Print and shaded views of the part. All mm, measured from the part's lowest x, y and z. A direction names the side the tool comes from. Round coordinates to 2 decimals unless told otherwise and drop trailing zeros. Loops run counter-clockwise (first coordinate to the right, second up) from the corner with the lowest first, then second, coordinate; pieces in that order, holes last. Notation, with made-up numbers: (-35, 27.5) - (1, 27.5) arc R19 ccw to (1, 57.5) - close; hole circle Ø2 at (83, 43). An arc over 180 degrees is marked (long way). Put each result on its own line as item: value. Start each with the question number.
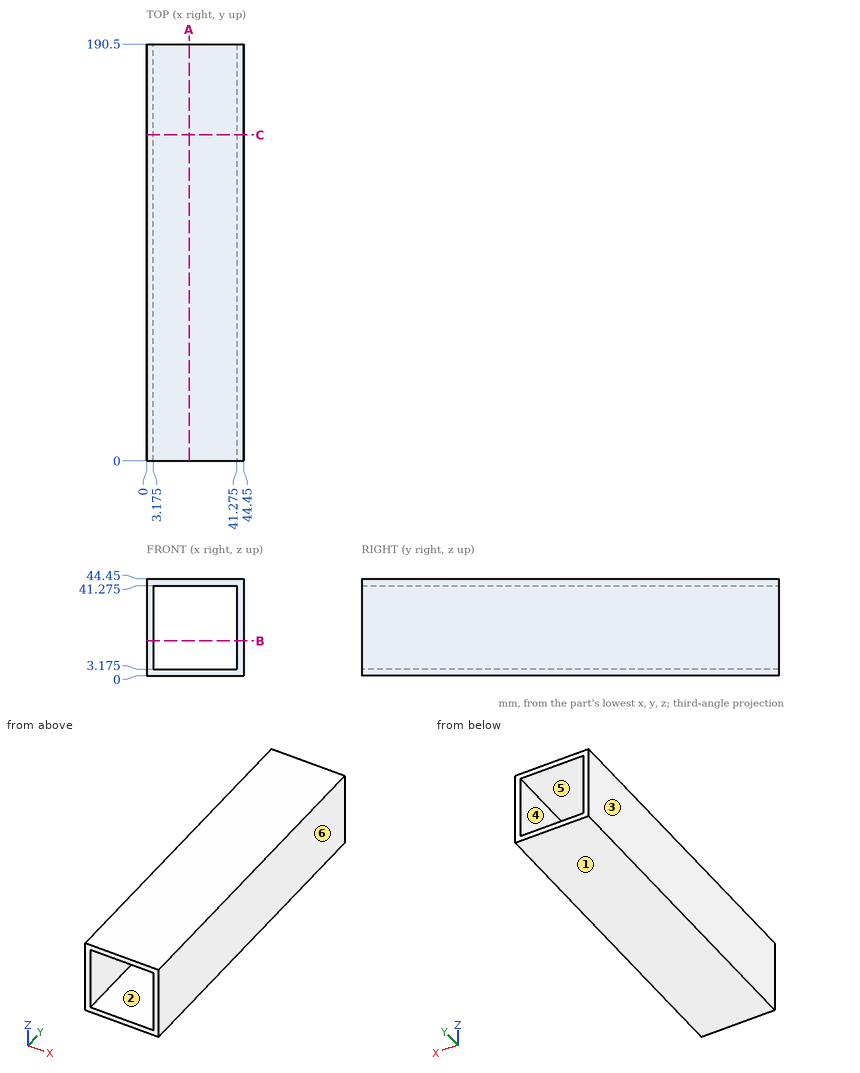
Item 1: Drop a flat-ended pin along its axis: pin 1 Ø3 at (x, z) = (21, 39) entering from +Y. Give the stop position or say it passes through.
Item 2: Which spindle directions (+Z, -Z, +X, -X, +Y, -Y) get a long thin tool onto all of the face, cutting with end or side? Do the marked faces 1 and 2. Say none if no direction does.
Item 3: Slice it at A-A (x = 19.5). Give the cut face in (y, z) (3 decimals), plus the area to 3 significant figures.
Item 4: Slice it at B-B (z = 16). Give the cut face in (x, y) (3 decimals).
Item 5: Drill centre line: probe 1 along Z at (x, y) = (34, 56) (3 decimals). Where is it in solid material? Low to high. Write a range as [from, to].
Item 6: Two-plate mould, pull along X, no slides. Class the marked faces 3, 4, 5 and 6: pulls with the +X half, pulls with the -X half, needs draft (parallel to the pull), parting line crosses it, or undercut.
Item 7: Slice it at C-C (y = 149). Give the cut face in (x, z) (3 decimals), plus the area to 3 significant figures.
Computed values:
1. pin 1: passes through
2. face 1: -Z, +X, -X, +Y, -Y
2. face 2: +Y, -Y
3. outline: (0, 0) - (190.5, 0) - (190.5, 3.175) - (0, 3.175) - close; (0, 41.275) - (190.5, 41.275) - (190.5, 44.45) - (0, 44.45) - close
3. area: 1,210 mm^2
4. outline: (0, 0) - (3.175, 0) - (3.175, 190.5) - (0, 190.5) - close; (41.275, 0) - (44.45, 0) - (44.45, 190.5) - (41.275, 190.5) - close
5. probe 1: z = [0, 3.175], [41.275, 44.45]
6. face 3: pulls with the -X half
6. face 4: undercut
6. face 5: undercut
6. face 6: pulls with the +X half
7. outline: (0, 0) - (44.45, 0) - (44.45, 44.45) - (0, 44.45) - close; hole (3.175, 3.175) - (41.275, 3.175) - (41.275, 41.275) - (3.175, 41.275) - close
7. area: 524 mm^2
